from build123d import *

# Parameters (mm, degrees)
F1_DEPTH     = 90
F3_R         = 7
F4_DEPTH     = 9
F5_R         = 3.35
F6_DEPTH     = 6
F7_SIZE      = 1
F8_R         = 3
F9_T1_DEPTH  = 84
F9_T3_DEPTH  = 24.1197014907
F9_T8_DEPTH  = 3
F9_T14_DEPTH = 3
F9_T20_DEPTH = 3
F9_T26_DEPTH = 3


# Not quite as in the source:
# - a fillet or chamfer that OpenCascade refuses, or shapes differently, is made with other operations: its cross-section is extruded or revolved along the edge and cut away or added


with BuildPart() as f1:
    # F0 (on Right) → F1 (new body)
    with BuildSketch(Plane.YZ):
        Polygon((-15, 6), (-15, 0), (15, 0), (15, 3), align=None)
    extrude(amount=F1_DEPTH)

    # F3 (on face) → F4 (join)
    with BuildSketch(Plane(origin=(0, 0, 0), x_dir=(1, 0, 0), z_dir=(0, 0, -1))):
        with Locations((70, 0)):
            Circle(F3_R)
        with Locations((20, 0)):
            Circle(F3_R)
    extrude(amount=F4_DEPTH)

    # F5 (on face) → F6 (cut)
    with BuildSketch(Plane(origin=(0, 0, -9), x_dir=(1, 0, 0), z_dir=(0, 0, -1))):
        with Locations((70, 0)):
            Circle(F5_R)
        with Locations((20, 0)):
            Circle(F5_R)
    extrude(amount=-F6_DEPTH, mode=Mode.SUBTRACT)

    # F7
    f7_edges = [f1.edges().sort_by_distance(p)[0] for p in [
        (63, 0, -9),
        (13, 0, -9),
    ]]
    chamfer(f7_edges, length=F7_SIZE)

    # F8
    f8_edges = [f1.edges().sort_by_distance(p)[0] for p in [
        (90, 15, 1.5),
        (0, 15, 1.5),
        (0, -15, 3),
        (90, -15, 3),
    ]]
    fillet(f8_edges, radius=F8_R)

    # F9: fillet of radius 3 on 4 edges, made by hand

    # F9_s2 → F9_t1 (cut)
    with BuildSketch(Plane.YZ.offset(3)):
        with BuildLine():
            ThreePointArc((15, 0.2850373137), (14.2243576007, 2.2980532759), (12.2985111571, 3.2701488843))
            Line((12.2985111571, 3.2701488843), (15, 3))
            Line((15, 3), (15, 0.2850373137))
        make_face()
        with BuildLine():
            ThreePointArc((-15, 2.6850373137), (-14.0130159623, 4.9093949143), (-11.7014888429, 5.6701488843))
            Line((-11.7014888429, 5.6701488843), (-15, 6))
            Line((-15, 6), (-15, 2.6850373137))
        make_face()
    extrude(amount=F9_T1_DEPTH, mode=Mode.SUBTRACT)

    # F9_s4 → F9_t3 (cut)
    with BuildSketch(Plane(origin=(0, 11.8529666026, -1.1852966603), x_dir=(1, 0, 0), z_dir=(0, -0.9950371902, 0.099503719))):
        with BuildLine():
            ThreePointArc((0, 1.4776673559), (0.8786796564, 3.5989876995), (3, 4.4776673559))
            Line((3, 4.4776673559), (0, 4.4776673559))
            Line((0, 4.4776673559), (0, 1.4776673559))
        make_face()
        with BuildLine():
            ThreePointArc((90, 1.4776673559), (89.1213203436, 3.5989876995), (87, 4.4776673559))
            Line((87, 4.4776673559), (90, 4.4776673559))
            Line((90, 4.4776673559), (90, 1.4776673559))
        make_face()
    extrude(amount=F9_T3_DEPTH, mode=Mode.SUBTRACT)


with BuildPart() as f9_tool6:
    # F9_s7 → F9_t8 (new body)
    with BuildSketch(Plane.YZ.offset(87)):
        Polygon((12, 0.2850373137), (15, 0.2850373137), (15, 3), (12.2985111571, 3.2701488843), align=None)
    extrude(amount=F9_T8_DEPTH)

    # F9_s9 → F9_t10 (revolve, cut)
    with BuildSketch(Plane(origin=(87, 12, 0.2850373137), x_dir=(0, -0.7414525336, -0.6710053208), z_dir=(0, -0.6710053208, 0.7414525336))):
        with BuildLine():
            ThreePointArc((0, -3), (3, 0), (0, 3))
            Line((0, 3), (0, -3))
        make_face()
    revolve(axis=Axis((87, 12, 0.2850373137), (1, 0, 0)), mode=Mode.SUBTRACT)


with BuildPart() as f1_1:
    add(f1.part)

    # F9_t5: cut F9_tool6
    add(f9_tool6.part, mode=Mode.SUBTRACT)


with BuildPart() as f9_tool12:
    # F9_s13 → F9_t14 (new body)
    with BuildSketch(Plane.YZ.offset(87)):
        Polygon((-12, 2.6850373137), (-15, 2.6850373137), (-15, 6), (-11.7014888429, 5.6701488843), align=None)
    extrude(amount=F9_T14_DEPTH)

    # F9_s15 → F9_t16 (revolve, cut)
    with BuildSketch(Plane(origin=(87, -12, 2.6850373137), x_dir=(0, 0.6710053208, -0.7414525336), z_dir=(0, -0.7414525336, -0.6710053208))):
        with BuildLine():
            ThreePointArc((0, -3), (3, 0), (0, 3))
            Line((0, 3), (0, -3))
        make_face()
    revolve(axis=Axis((87, -12, 2.6850373137), (1, 0, 0)), mode=Mode.SUBTRACT)


with BuildPart() as f1_2:
    add(f1_1.part)

    # F9_t11: cut F9_tool12
    add(f9_tool12.part, mode=Mode.SUBTRACT)


with BuildPart() as f9_tool18:
    # F9_s19 → F9_t20 (new body)
    with BuildSketch(Plane.YZ.offset(3)):
        Polygon((12, 0.2850373137), (15, 0.2850373137), (15, 3), (12.2985111571, 3.2701488843), align=None)
    extrude(amount=-F9_T20_DEPTH)

    # F9_s21 → F9_t22 (revolve, cut)
    with BuildSketch(Plane(origin=(3, 12, 0.2850373137), x_dir=(0, -0.7414525336, -0.6710053208), z_dir=(0, 0.6710053208, -0.7414525336))):
        with BuildLine():
            ThreePointArc((0, -3), (3, 0), (0, 3))
            Line((0, 3), (0, -3))
        make_face()
    revolve(axis=Axis((3, 12, 0.2850373137), (-1, 0, 0)), mode=Mode.SUBTRACT)


with BuildPart() as f1_3:
    add(f1_2.part)

    # F9_t17: cut F9_tool18
    add(f9_tool18.part, mode=Mode.SUBTRACT)


with BuildPart() as f9_tool24:
    # F9_s25 → F9_t26 (new body)
    with BuildSketch(Plane.YZ.offset(3)):
        Polygon((-12, 2.6850373137), (-15, 2.6850373137), (-15, 6), (-11.7014888429, 5.6701488843), align=None)
    extrude(amount=-F9_T26_DEPTH)

    # F9_s27 → F9_t28 (revolve, cut)
    with BuildSketch(Plane(origin=(3, -12, 2.6850373137), x_dir=(0, 0.6710053208, -0.7414525336), z_dir=(0, 0.7414525336, 0.6710053208))):
        with BuildLine():
            ThreePointArc((0, -3), (3, 0), (0, 3))
            Line((0, 3), (0, -3))
        make_face()
    revolve(axis=Axis((3, -12, 2.6850373137), (-1, 0, 0)), mode=Mode.SUBTRACT)


with BuildPart() as f1_4:
    add(f1_3.part)

    # F9_t23: cut F9_tool24
    add(f9_tool24.part, mode=Mode.SUBTRACT)


solid = f1_4.part
Could you check a few things on this model? Use its own coordinates, in mm. A direction names the side the tool comes from. Give positions to 0.01 mm unless a question says otherwise; leave off trailing zeros. Order: outer loops, then holes, each group sorted by start corner. A loop starts at its lowest first (then second) coordinate and runs counter-clockwise, first axis right, second up. Notation, with made-up numbers: (71.5, 70) -> (125.5, 70) arc R19 ccw to (125.5, 105) -> close; hole circle Ø11 at (-22, 75.5). An arc over 180 degrees is marked (long way). Answer in a Markdown table with one row per item. Add a question column.
Item 1: I'm going to push flat-ended pins straight in: P1, Ø1.5, axis at y = -5.5, z = -6.5, coming from the -X side; P2, Ø8.5, axis at x = 20, y = 0, coming from the +Z side (3 decimals); P3, Ø2, axis at x = 61, z = -2.5, coming from the -Y side; P4, Ø2, axis at x = 70, y = -0.5, coming from the -Z side. Where does each tip first touch, or does it pass through?
Item 2: Please list where these lines run through material, in increasing order: probe 1 along X at (y, z) = (0, -7.3); probe 2 along Y at (x, z) = (70, -5.05); probe 3 along X at (y, z) = (6.25, -7.5).
Item 3: Imagine slicing it at B-B (x = 70). List the corners of the cut face in (y, z) for me, and give its area (3 significant figures).
Item 4: Imagine slicing it at C-C (x = 12). List the corners of the cut face in (y, z) for me, and give its area (3 significant figures).
Item 5: Imagine slicing it at A-A (z = -4.25). List the corners of the cut face in (x, y) for me.
Item 6: We'd pull the mould along X, two halves only. Please class faces 1 (the cylindrical face through (64.445, 4.259, -3.944)), 2 (the cylindrical face through (44.412, -14.039, 4.886)), 3 (the flat face through (0, -3, 1)): pulls with the +X half, pulls with the -X half, needs draft (parallel to the pull), parting line crosses it, or undercut.
Item 7: For faces 4 (the flat face through (73, 3, -9)), 5 (the flat face through (44, 0, 0)), which set-ups out of +Z, -Z, +X, -X, +Y, -Y let a thin tool reach every point of the face, with its end or its side?
Result:
| question | item | result |
|---|---|---|
| 1 | P1 | x = 14.86 |
| 1 | P2 | z = 4.925 |
| 1 | P3 | through |
| 1 | P4 | z = -3 |
| 2 | probe 1 | 13 to 16.65, 23.35 to 27, 63 to 66.65, 73.35 to 77 |
| 2 | probe 2 | -7 to -3.35, 3.35 to 7 |
| 2 | probe 3 | 16.85 to 23.15, 66.85 to 73.15 |
| 3 | outline | (-15, 0) -> (-7, 0) -> (-7, -8) -> (-6, -9) -> (-3.35, -9) -> (-3.35, -3) -> (3.35, -3) -> (3.35, -9) -> (6, -9) -> (7, -8) -> (7, 0) -> (15, 0) -> (15, 0.29) arc R3 ccw to (12.3, 3.27) -> (-11.7, 5.67) arc R3 ccw to (-15, 2.69) -> close |
| 3 | area | 216 mm2 |
| 4 | outline | (-15, 0) -> (15, 0) -> (15, 0.29) arc R3 ccw to (12.3, 3.27) -> (-11.7, 5.67) arc R3 ccw to (-15, 2.69) -> close |
| 4 | area | 131 mm2 |
| 5 | outline | circle Ø14 at (20, 0); circle Ø14 at (70, 0); hole circle Ø6.7 at (20, 0); hole circle Ø6.7 at (70, 0) |
| 6 | face 1 | undercut |
| 6 | face 2 | needs draft |
| 6 | face 3 | pulls with the -X half |
| 7 | face 4 | -Z, +X, -X, +Y, -Y |
| 7 | face 5 | -Z |
